Source: CAD feature listing. Evaluate the final solid. Frame: model axes, mm. Face numbers are marked on the shaded views. A direction names the side the tool comes from. Give positions to 0.01 mm unless a question says otherwise; leave off trailing zeros. Loops run counter-clockwise (first coordinate to the right, second up) from the corner with the lowest first, then second, coordinate; pieces in that order, holes last. Notation, with made-up numbers: (20.5, 4) - (74.5, 4) arc R32 ccw to (74.5, 30) - close; hole circle Ø6 at (27.5, 87). An arc over 180 degrees is marked (long way). Put each result on its own line as item: value.
Autodesk Inventor part; units mm, degrees
ref_plane "YZ Plane" through (0, 0, 0) normal (1, 0, 0) x (0, 1, 0)
ref_plane "XZ Plane" through (0, 0, 0) normal (0, 1, 0) x (-1, 0, 0)
ref_plane "XY Plane" through (0, 0, 0) normal (0, 0, 1) x (1, 0, 0)
sketch "Sketch1" plane through (0, 0, 0) normal (0, 1, 0) x (-1, 0, 0)
  circle A0 centre (0, 0) radius 10.0965
  dimension "d0" = 20.193
extrude "Extrusion1" add sketch "Sketch1" along normal blind 25.4
sketch "Sketch2" plane through (0, 25.4, 0) normal (0, 1, 0) x (1, 0, 0)
  circle A0 centre (0, 0) radius 10.0965
  circle A1 centre (0, 0) radius 38.1
  dimension "d3" = 76.2
extrude "Extrusion2" add sketch "Sketch2" along normal blind 50.8
loft "Loft1" add section 1 edges at (10.0965, 0, 0) section 2 edges at (-38.1, 25.4, 0)
fillet "Fillet1" radius 3.175 2 edges at (0, 25.4, -38.1) (0, 25.4, 38.1)
sketch "Sketch3" plane through (0, 25.4, 0) normal (0, 1, 0) x (1, 0, 0)
  circle A0 centre (0, 0) radius 10.0965
  circle A1 centre (0, 0) radius 10.0965
extrude "Extrusion3" add sketch "Sketch3" along normal blind 50.8
shell "Shell1" thickness 2.54 removed faces 1 at (18.352, 76.2, 0)
sketch "Sketch4" plane through (0, 0, 0) normal (0, -1, 0) x (1, 0, 0)
  circle A0 centre (0, 0) radius 10.0965
  circle A1 centre (0, 0) radius 8.8265
  dimension "d14" = 17.653
extrude "Extrusion4" cut sketch "Sketch4" against normal blind 50.8 contours A1
sketch "Sketch5" plane through (0, 0, 0) normal (0, -1, 0) x (1, 0, 0)
  circle A0 centre (0, 0) radius 8.8265
  circle A1 centre (0, 0) radius 10.0965
  circle A2 centre (0, 0) radius 8.8265
  circle A3 centre (0, 0) radius 10.0965
extrude "Extrusion5" add sketch "Sketch5" along normal blind 7.62
properties part number "Hopper"
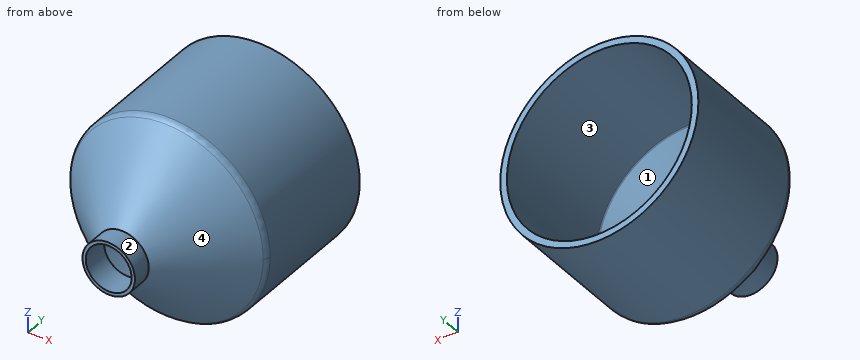
1) Material intervals for line 1 along X through (y, z) = (49.5, 0); line 2 along Z through (x, y) = (7, 37); line 3 along X through (y, z) = (15.5, -6.5), sorted ascending. Write a range as [from, to].
Check result:
line 1: [-38.1, -35.56], [35.56, 38.1]
line 2: [-37.45, -34.86], [34.86, 37.45]
line 3: [-26.4, -22.48], [22.48, 26.4]
2) Pin query (flat end, axial travel): P1, Ø12, axis at x = 12, z = -27.5, coming from the -Y side; P2, Ø5.5, axis at x = 3, z = -3.5, coming from the +Y side; P3, Ø5, axis at y = 31.5, z = 9.5, coming from the +X side; P4, Ø3, axis at x = -26.5, y = 30, coming from the -Z side. Return the tip coordinate at first contact, or that it passes through.
Check result:
P1: y = 12.61
P2: through
P3: x = 37.45
P4: z = -28.75
3) Section query A-A, the plane y = 44. Output: boundary loops of the cut face in (x, z), plus the area to 3 significant figures.
Check result:
outline: circle Ø76.2 at (0, 0); hole circle Ø71.12 at (0, 0)
area: 588 mm²
4) Mould query, pull axis X, two halves, no side actions, for the marked faces 1 and 2. Classes: pulls with the +X half, pulls with the -X half, needs draft (parallel to the pull), parting line crosses it, or undercut.
Check result:
face 1: undercut
face 2: parting line crosses it
5) Section query B-B, the plane y = 22.5. Output: boundary loops of the cut face in (x, z), plus the area to 3 significant figures.
Check result:
outline: circle Ø69.81 at (0, 0); hole circle Ø62.24 at (0, 0)
area: 784 mm²
6) Access query for the marked faces 3 and 4. Directions: +Z, -Z, +X, -X, +Y, -Y. A direction counts if a zero-diameter tool reaches every point of the face in a straight line with its end or side. Return the directions, or none.
Check result:
face 3: +Y
face 4: -Y
